from build123d import *

# Parameters (mm, degrees)
SALIENTE_EXTRUIR1_DEPTH = 7.5
CROQUIS2_R              = 1.25
SALIENTE_EXTRUIR2_DEPTH = 2
SALIENTE_EXTRUIR3_DEPTH = 7


with BuildPart() as part:
    # Croquis1 → Saliente-Extruir1 (new body)
    with BuildSketch(Plane.XY):
        Polygon((-8.919750427, 0), (8.919750427, 0), (16.419750427, -12.990381057), (-16.419750427, -12.990381057), align=None)
    extrude(amount=SALIENTE_EXTRUIR1_DEPTH)

    # Croquis2 → Saliente-Extruir2 (add)
    with BuildSketch(Plane.XY.offset(7.5)):
        Polygon((-8.919750427, 0), (-16.419750427, 4.330127019), (-18.59607878, 3.240107663), (-30.143084163, 3.240107663), (-33.029835509, -1.759892337), (-15.709327434, -11.759892337), (-16.419750427, -12.990381057), (16.419750427, -12.990381057), (15.709327434, -11.759892337), (33.029835509, -1.759892337), (30.143084163, 3.240107663), (18.59607878, 3.240107663), (16.419750427, 4.330127019), (8.919750427, 0), align=None)
        with Locations((-26.726205798, -0.841685406)):
            Circle(CROQUIS2_R, mode=Mode.SUBTRACT)
        with Locations((-18.498964463, -5.591685406)):
            Circle(CROQUIS2_R, mode=Mode.SUBTRACT)
        with Locations((18.498964463, -5.591685406)):
            Circle(CROQUIS2_R, mode=Mode.SUBTRACT)
        with Locations((26.726205798, -0.841685406)):
            Circle(CROQUIS2_R, mode=Mode.SUBTRACT)
    extrude(amount=SALIENTE_EXTRUIR2_DEPTH)

    # Croquis3 → Saliente-Extruir3 (add)
    with BuildSketch(Plane(origin=(0, 0, 7.5), x_dir=(-1, 0, 0), z_dir=(0, 0, -1))):
        Polygon((-18.549679438, 3.263346886), (-16.419750427, 4.330127019), (-8.919750427, 0), (-9.914162027, -1.722371415), align=None)
        Polygon((-30.305258965, -3.332927338), (-24.369581471, -6.759892337), (-23.490602897, -5.237456788), (-26.081610625, -3.741537779), (-26.729742931, -3.993881902), (-29.396625899, -2.454156302), (-29.711298573, -1.645936465), (-30.590277147, -3.168372014), align=None)
        Polygon((-21.307825634, -8.527597894), (-20.660765693, -7.4068572), (-18.160959134, -8.850121189), (-18.808019075, -9.970861884), align=None)
        Polygon((9.914162027, -1.722371415), (18.549679438, 3.263346886), (16.419750427, 4.330127019), (8.919750427, 0), align=None)
        Polygon((18.160959134, -8.850121189), (18.808019075, -9.970861884), (21.307825634, -8.527597894), (20.660765693, -7.4068572), align=None)
        Polygon((29.711298573, -1.645936465), (30.590277147, -3.168372014), (30.305258965, -3.332927338), (24.369581471, -6.759892337), (23.490602897, -5.237456788), (26.081610625, -3.741537779), (26.729742931, -3.993881902), (29.396625899, -2.454156302), align=None)
    extrude(amount=SALIENTE_EXTRUIR3_DEPTH)


solid = part.part
Verification items for the finished model (mm, model axes). A direction names the side the tool comes from. Coordinates: 2 decimals unless noted, no trailing zeros. Write each loop counter-clockwise with the first axis right and the second up, starting at its lowest first coordinate (ties: lowest second). Pieces come first, ordered by that corner, then holes. Notation, with made-up numbers: (71, 63.5) -> (112, 63.5) arc R28 ccw to (112, 81.5) -> close; hole circle Ø7 at (54.25, -30.75). An arc over 180 degrees is marked (long way). One line per item, written item: value. Start each with the question number.
Q1. Cross-section at B-B on y = 1.5. Enter the section's corners in (x, z), and give its area (3 significant figures).
Q2. Mould release check, pull along X, two halves, no side actions. Record for faces 1 (the flat face through (-13, 2, 0.5)), 2 (the flat face through (-12.617, 2.135, 4.937)), 3 (the flat face through (-20.99, -7.98, 4.05)): pulls with the +X half, pulls with the -X half, needs draft (parallel to the pull), parting line crosses it, or undercut.
Q3. Cross-section at A-A on z = 2. State how many separate pieces and enclosed holes the cut face has, and give its area (3 significant figures).
Q4. Access from +Z, -Z, +X, -X, +Y, -Y to the whole of each face (thin tool, end or side, straight path). Record for faces 4 (the flat face through (12.722, 2.195, 5.063)), 5 (the flat face through (-18.48, -9.4, 4.05)), 6 (the flat face through (20.99, -7.98, 4.05)), 7 (the flat face through (27.1, -4.4, 0.5)).
Q5. Go/stop test with flat-tipped pins: P1, Ø0.8, axis at x = 19, y = -8.5, coming from the -Z side; P2, Ø5, axis at y = -11, z = 8.5, coming from the -X side; P3, Ø1.5, axis at y = -1.5, z = 8, coming from the -X side; P4, Ø0.6, axis at x = 23.5, z = 9, coming from the +Y side. Record where each tip stops, or that it passes through.
Q6. Cross-section at C-C on x = 6. Enter the section's corners in (y, z).
Q7. Thickness scan on L1, parallel to X at y = -3.5, z = 1.75; L2, parallel to Z at x = 20, y = -1.75; L3, parallel to Y at x = -8.5, z = 6.5. Record the ranges inside material, lowest first. Write a range as from..to.
Checked values:
1. outline: (-31.15, 7.5) -> (-15.5, 7.5) -> (-15.5, 0.5) -> (-11.52, 0.5) -> (-11.52, 9.5) -> (-31.15, 9.5) -> close; (11.52, 0.5) -> (15.5, 0.5) -> (15.5, 7.5) -> (31.15, 7.5) -> (31.15, 9.5) -> (11.52, 9.5) -> close
1. area: 134 mm²
2. face 1: needs draft
2. face 2: undercut
2. face 3: pulls with the -X half
3. separate pieces: 5
3. enclosed holes: 0
3. area: 395 mm²
4. face 4: +Z, -Z, +Y
4. face 5: -Z, -Y
4. face 6: -Z, +X, +Y
4. face 7: -Z, +X, +Y, -Y
5. P1: stops at z = 0.5
5. P2: stops at x = -21.36
5. P3: stops at x = -33.03
5. P4: stops at y = 3.24
6. outline: (-12.99, 0) -> (0, 0) -> (0, 9.5) -> (-12.99, 9.5) -> close
7. L1: x = -30.02..-27.59, -10.94..10.94, 27.59..30.02
7. L2: z = 7.5..9.5
7. L3: y = -12.99..0
